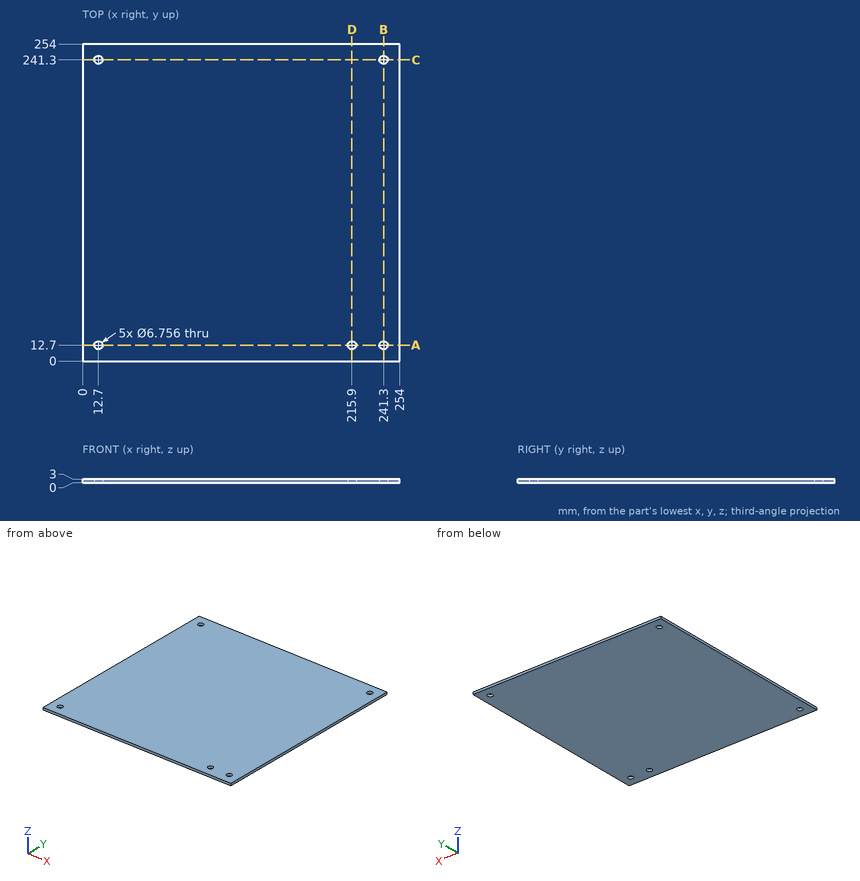
Source: three-view drawing plus pictorial views. Frame: mm from the lowest corner of the part. Round coordinates to 2 decimals unless told otherwise and drop trailing zeros. Order: outer loops, then holes, each group sorted by start corner. A loop starts at its lowest first (then second) coordinate and runs counter-clockwise, first axis right, second up. Notation, with made-up numbers: (-26.5, -10.5) - (-1.5, -10.5) arc R17 ccw to (-1.5, -2.5) - close; hole circle Ø2 at (-32.5, 81). An arc over 180 degrees is marked (long way). Answer in a Markdown table with one row per item.
Item 1: Line query: line 1 (X direction, y = 12.7, z = 1.65); line 2 (Y direction, x = 241.3, z = 0.9). Output: solid intervals per line, ascending.
Model answer:
| item | result |
|---|---|
| line 1 | x = 0 to 9.32, 16.08 to 212.52, 219.28 to 237.92, 244.68 to 254 |
| line 2 | y = 0 to 9.32, 16.08 to 237.92, 244.68 to 254 |
Item 2: Section query B-B (x = 241.3). Return the cut outline in (y, z).
Model answer:
| item | result |
|---|---|
| outline | (0, 0) - (9.32, 0) - (9.32, 3) - (0, 3) - close; (16.08, 0) - (237.92, 0) - (237.92, 3) - (16.08, 3) - close; (244.68, 0) - (254, 0) - (254, 3) - (244.68, 3) - close |
Item 3: Section query D-D (x = 215.9). Return the cut outline in (y, z).
Model answer:
| item | result |
|---|---|
| outline | (0, 0) - (9.32, 0) - (9.32, 3) - (0, 3) - close; (16.08, 0) - (254, 0) - (254, 3) - (16.08, 3) - close |
Item 4: Pin query (flat end, axial travel): pin 1 (1.5 mm diameter, centred on x = 173, z = 1.5, fed in from -Y). Return the tip coordinate at first contact, or that it passes through.
Model answer:
| item | result |
|---|---|
| pin 1 | stops at y = 0 |
Item 5: Section query A-A (y = 12.7). Return the cut outline in (x, z).
Model answer:
| item | result |
|---|---|
| outline | (0, 0) - (9.32, 0) - (9.32, 3) - (0, 3) - close; (16.08, 0) - (212.52, 0) - (212.52, 3) - (16.08, 3) - close; (219.28, 0) - (237.92, 0) - (237.92, 3) - (219.28, 3) - close; (244.68, 0) - (254, 0) - (254, 3) - (244.68, 3) - close |
